from build123d import *

# Parameters (mm, degrees)
SKETCH2_W           = 365
SKETCH2_H           = 188
BOSS_EXTRUDE1_DEPTH = 272
SKETCH3_W           = 345.774876004
SKETCH3_H           = 174.045166382
BOSS_EXTRUDE2_DEPTH = 10
BOSS_EXTRUDE3_DEPTH = 10
SKETCH5_R           = 15.372297264
SKETCH5_R_2         = 15.186201359
BOSS_EXTRUDE4_DEPTH = 4


with BuildPart() as part:
    # Sketch2 → Boss-Extrude1 (new body)
    with BuildSketch(Plane.XY):
        Rectangle(SKETCH2_W, SKETCH2_H)
    extrude(amount=BOSS_EXTRUDE1_DEPTH)

    # Sketch3 → Boss-Extrude2 (add)
    with BuildSketch(Plane.XY.offset(272)):
        Rectangle(SKETCH3_W, SKETCH3_H)
    extrude(amount=BOSS_EXTRUDE2_DEPTH)

    # Sketch4 → Boss-Extrude3 (add)
    with BuildSketch(Plane.XY.offset(282)):
        Polygon((146.126879862, 56.64254241), (141.134054035, 65.290370416), (131.14840238, 65.290370416), (126.155576553, 56.64254241), (131.14840238, 47.994714404), (141.134054035, 47.994714404), align=None)
        Polygon((146.126879862, -52.289546401), (141.134054035, -43.641718394), (131.14840238, -43.641718394), (126.155576553, -52.289546401), (131.14840238, -60.937374407), (141.134054035, -60.937374407), align=None)
    extrude(amount=BOSS_EXTRUDE3_DEPTH)

    # Sketch5 → Boss-Extrude4 (add)
    with BuildSketch(Plane.XY.offset(282)):
        with Locations((136.141228208, 56.003971115)):
            Circle(SKETCH5_R)
        with Locations((136.141228208, -52.041649492)):
            Circle(SKETCH5_R_2)
    extrude(amount=BOSS_EXTRUDE4_DEPTH)


solid = part.part
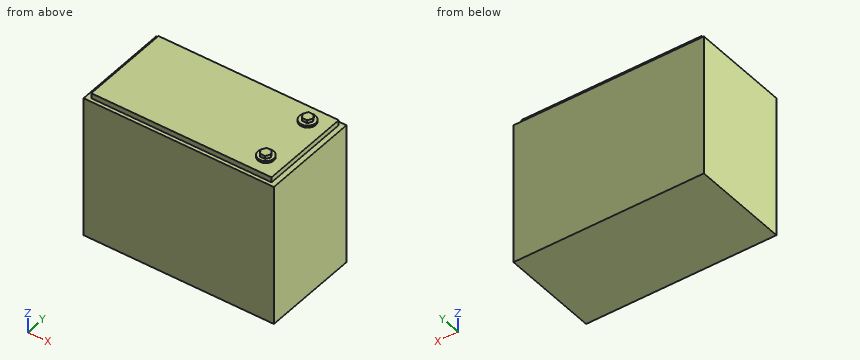
For this review, take the finished solid that the model builds, in its own axes (mm). Round coordinates to 2 decimals unless told otherwise and drop trailing zeros. Loops run counter-clockwise (first coordinate to the right, second up) from the corner with the lowest first, then second, coordinate; pieces in that order, holes last. Notation, with made-up numbers: (35.5, 36) - (40.5, 36) arc R10 cw to (40.5, 51) - close; hole circle Ø6 at (-5, 89). An arc over 180 degrees is marked (long way). One line per question, with ' | ' between items.
Q1. For pin 1 (3 mm diameter, centred on x = 135, z = 289, fed in from -Y); pin 2 (3 mm diameter, centred on x = 137.5, z = 290, fed in from +Y); pin 3 (4 mm diameter, centred on x = -146, y = 35, fed in from +Z), all flat-tipped, find the tip position at first contact; note any pin that passes through.
Taken from the geometry:
pin 1: stops at y = -60.94 | pin 2: stops at y = 65.29 | pin 3: stops at z = 282
Q2. For line 1 along Z through (x, y) = (49, -51), list the stretches that pass through material, from the lowest coordinate up. Write a range as [from, to].
Taken from the geometry:
line 1: z = [0, 282]
Q3. Take a section at A-A (y = -17). Give the boundary of the cut face in (x, z), and give its area (3 significant figures).
Taken from the geometry:
outline: (-182.5, 0) - (182.5, 0) - (182.5, 272) - (172.89, 272) - (172.89, 282) - (-172.89, 282) - (-172.89, 272) - (-182.5, 272) - close | area: 103,000 mm²
Q4. Take a section at B-B (x = 34.5). Give the boundary of the cut face in (y, z).
Taken from the geometry:
outline: (-94, 0) - (94, 0) - (94, 272) - (87.02, 272) - (87.02, 282) - (-87.02, 282) - (-87.02, 272) - (-94, 272) - close
